from build123d import *

# Parameters (mm, degrees)
F0_R     = 11
F1_DEPTH = 7


with BuildPart() as f1:
    # F0 (on Top) → F1 (new body)
    with BuildSketch(Plane.XY):
        with BuildLine():
            ThreePointArc((-10.362367, 34.413892), (-13.196178, 29.675563), (-13.977698, 24.210082))
            ThreePointArc((-13.977698, 24.210082), (-24.891005, 26.119838), (-33.774991, 19.5))
            ThreePointArc((-33.774991, 19.5), (-35.570661, 13.994279), (-34.984488, 8.232873))
            ThreePointArc((-34.984488, 8.232873), (-32.29788, 3.409556), (-27.955395, 0))
            ThreePointArc((-27.955395, 0), (-35.065946, -8.496324), (-33.774991, -19.5))
            ThreePointArc((-33.774991, -19.5), (-29.904732, -23.807957), (-24.622121, -26.181019))
            ThreePointArc((-24.622121, -26.181019), (-19.101702, -26.266007), (-13.977698, -24.210082))
            ThreePointArc((-13.977698, -24.210082), (-10.174941, -34.616162), (0, -39))
            ThreePointArc((0, -39), (5.665929, -37.802236), (10.362367, -34.413892))
            ThreePointArc((10.362367, -34.413892), (13.196178, -29.675563), (13.977698, -24.210082))
            ThreePointArc((13.977698, -24.210082), (24.891005, -26.119838), (33.774991, -19.5))
            ThreePointArc((33.774991, -19.5), (35.570661, -13.994279), (34.984488, -8.232873))
            ThreePointArc((34.984488, -8.232873), (32.29788, -3.409556), (27.955395, 0))
            ThreePointArc((27.955395, 0), (35.065946, 8.496324), (33.774991, 19.5))
            ThreePointArc((33.774991, 19.5), (29.904732, 23.807957), (24.622121, 26.181019))
            ThreePointArc((24.622121, 26.181019), (19.101702, 26.266007), (13.977698, 24.210082))
            ThreePointArc((13.977698, 24.210082), (10.174941, 34.616162), (0, 39))
            ThreePointArc((0, 39), (-5.665929, 37.802236), (-10.362367, 34.413892))
        make_face()
        with Locations((-21.650635, -12.5)):
            Circle(F0_R, mode=Mode.SUBTRACT)
        with BuildLine():
            ThreePointArc((-6.30476, -12.5), (-7, -12.875644), (-7.672937, -13.289918))
            ThreePointArc((-7.672937, -13.289918), (-7.650635, -12.5), (-7.672937, -11.710082))
            ThreePointArc((-7.672937, -11.710082), (-7, -12.124356), (-6.30476, -12.5))
        make_face(mode=Mode.SUBTRACT)
        with Locations((0, -25)):
            Circle(F0_R, mode=Mode.SUBTRACT)
        with BuildLine():
            ThreePointArc((7.672937, -11.710082), (7.650635, -12.5), (7.672937, -13.289918))
            ThreePointArc((7.672937, -13.289918), (7, -12.875644), (6.30476, -12.5))
            ThreePointArc((6.30476, -12.5), (7, -12.124356), (7.672937, -11.710082))
        make_face(mode=Mode.SUBTRACT)
        with Locations((21.650635, -12.5)):
            Circle(F0_R, mode=Mode.SUBTRACT)
        with Locations((-21.650635, 12.5)):
            Circle(F0_R, mode=Mode.SUBTRACT)
        with BuildLine():
            ThreePointArc((-15.345875, 0), (-14.650635, 0.375644), (-13.977698, 0.789918))
            ThreePointArc((-13.977698, 0.789918), (-14, 0), (-13.977698, -0.789918))
            ThreePointArc((-13.977698, -0.789918), (-14.650635, -0.375644), (-15.345875, 0))
        make_face(mode=Mode.SUBTRACT)
        with BuildLine():
            ThreePointArc((-7.672937, 11.710082), (-7.650635, 12.5), (-7.672937, 13.289918))
            ThreePointArc((-7.672937, 13.289918), (-7, 12.875644), (-6.30476, 12.5))
            ThreePointArc((-6.30476, 12.5), (-7, 12.124356), (-7.672937, 11.710082))
        make_face(mode=Mode.SUBTRACT)
        Circle(F0_R, mode=Mode.SUBTRACT)
        with BuildLine():
            ThreePointArc((13.977698, -0.789918), (14, 0), (13.977698, 0.789918))
            ThreePointArc((13.977698, 0.789918), (14.650635, 0.375644), (15.345875, 0))
            ThreePointArc((15.345875, 0), (14.650635, -0.375644), (13.977698, -0.789918))
        make_face(mode=Mode.SUBTRACT)
        with BuildLine():
            ThreePointArc((6.30476, 12.5), (7, 12.875644), (7.672937, 13.289918))
            ThreePointArc((7.672937, 13.289918), (7.650635, 12.5), (7.672937, 11.710082))
            ThreePointArc((7.672937, 11.710082), (7, 12.124356), (6.30476, 12.5))
        make_face(mode=Mode.SUBTRACT)
        with Locations((21.650635, 12.5)):
            Circle(F0_R, mode=Mode.SUBTRACT)
        with Locations((0, 25)):
            Circle(F0_R, mode=Mode.SUBTRACT)
        with BuildLine():
            ThreePointArc((-34.984488, 8.232873), (-35.570661, 13.994279), (-33.774991, 19.5))
            Line((-33.774991, 19.5), (-40.018085, 8.686644))
            ThreePointArc((-40.018085, 8.686644), (-39.972979, 8.121164), (-39.428556, 7.961773))
            ThreePointArc((-39.428556, 7.961773), (-37.224068, 8.384953), (-34.984488, 8.232873))
        make_face()
        with BuildLine():
            ThreePointArc((-12.81918, 38.127017), (-11.350452, 36.429465), (-10.362367, 34.413892))
            ThreePointArc((-10.362367, 34.413892), (-5.665929, 37.802236), (0, 39))
            Line((0, 39), (-12.486188, 39))
            ThreePointArc((-12.486188, 39), (-12.953356, 38.678197), (-12.81918, 38.127017))
        make_face()
        with BuildLine():
            ThreePointArc((-24.622121, -26.181019), (-29.904732, -23.807957), (-33.774991, -19.5))
            Line((-33.774991, -19.5), (-27.531897, -30.313356))
            ThreePointArc((-27.531897, -30.313356), (-27.019624, -30.557034), (-26.609375, -30.165244))
            ThreePointArc((-26.609375, -30.165244), (-25.873616, -28.044512), (-24.622121, -26.181019))
        make_face()
        with BuildLine():
            ThreePointArc((26.609375, 30.165244), (25.873616, 28.044512), (24.622121, 26.181019))
            ThreePointArc((24.622121, 26.181019), (29.904732, 23.807957), (33.774991, 19.5))
            Line((33.774991, 19.5), (27.531897, 30.313356))
            ThreePointArc((27.531897, 30.313356), (27.019624, 30.557034), (26.609375, 30.165244))
        make_face()
        with BuildLine():
            ThreePointArc((10.362367, -34.413892), (5.665929, -37.802236), (0, -39))
            Line((0, -39), (12.486188, -39))
            ThreePointArc((12.486188, -39), (12.953356, -38.678197), (12.81918, -38.127017))
            ThreePointArc((12.81918, -38.127017), (11.350452, -36.429465), (10.362367, -34.413892))
        make_face()
        with BuildLine():
            ThreePointArc((39.428556, -7.961773), (37.224068, -8.384953), (34.984488, -8.232873))
            ThreePointArc((34.984488, -8.232873), (35.570661, -13.994279), (33.774991, -19.5))
            Line((33.774991, -19.5), (40.018085, -8.686644))
            ThreePointArc((40.018085, -8.686644), (39.972979, -8.121164), (39.428556, -7.961773))
        make_face()
    extrude(amount=F1_DEPTH)


solid = f1.part
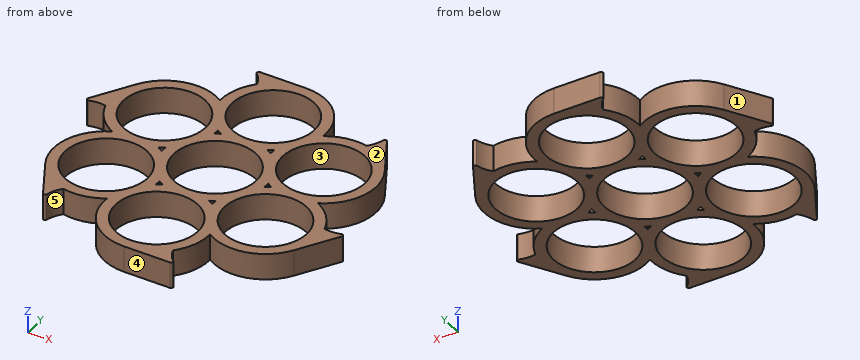
Model file for the job. Use its own axes, mm. Face numbers are marked on the shaded views. A direction names the side the tool comes from. Give positions to 0.01 mm unless a question says otherwise; leave off trailing zeros. Loops run counter-clockwise (first coordinate to the right, second up) from the corner with the lowest first, then second, coordinate; pieces in that order, holes last.
1) Pull direction Y, two halves, no side cores. Call the marked faces 1, 2 and 3: +Y half, -Y half, draft (parallel to the pull), parting line (faces both ways), or undercut.
2) Saw through at D-D (z = 1). Count the separate pieces of the cut face and the enclosed holes in it, plus the area to 3 significant figures.
3) Tool access for the marked faces 4 and 5: list every direction of +Z, -Z, +X, -X, +Y, -Y with a clear straight run to the whole face (end or side of a thin tool).
4) Saw through at A-A (x = -1). Write the cut outline in (y, z).
5) Flat gauge pins, fed straight in: pin 1 Ø17.5 at (x, y) = (21.65, -12.5) entering from -Z; pin 2 Ø2 at (y, z) = (19, 3.5) entering from +X (3 decimals). Where does each tip first touch, or does it go through?
6) Wall check: line 1 (X direction, y = -19.5, z = 3.5) (3 decimals); line 2 (Y direction, x = 3.5, z = 6.75); line 3 (X direction, y = -5, z = 2.5). Give the ranges that are in metal, low to high.
7) Saw through at B-B (x = 19). Write the cut outline in (y, z).
8) Saw through at C-C (y = -3.5). Write the cut outline in (x, z), plus the area to 3 significant figures.
Answer block:
1. face 1: +Y half
1. face 2: draft
1. face 3: undercut
2. separate pieces: 1
2. enclosed holes: 13
2. area: 1,470 mm2
3. face 4: +Z, -Z, +X, -X, -Y
3. face 5: +Z, -Z, -Y
4. outline: (-38.96, 0) - (-35.95, 0) - (-35.95, 7) - (-38.96, 7) - close; (-14.05, 0) - (-10.95, 0) - (-10.95, 7) - (-14.05, 7) - close; (10.95, 0) - (14.05, 0) - (14.05, 7) - (10.95, 7) - close; (35.95, 0) - (39, 0) - (39, 7) - (35.95, 7) - close
5. pin 1: passes through
5. pin 2: stops at x = 34.525
6. line 1: x = -33.775 to -30.136, -13.165 to -9.526, 9.526 to 13.165, 30.136 to 33.775
6. line 2: y = -39 to -35.43, -14.57 to -10.43, 10.43 to 14.57, 35.43 to 38.56
6. line 3: x = -33.47 to -29.7, -13.6 to -9.8, 9.8 to 13.6, 29.7 to 33.47
7. outline: (-26.25, 0) - (-23.18, 0) - (-23.18, 7) - (-26.25, 7) - close; (-1.82, 0) - (1.82, 0) - (1.82, 7) - (-1.82, 7) - close; (23.18, 0) - (26.25, 0) - (26.25, 7) - (23.18, 7) - close
8. outline: (-32.37, 0) - (-27.98, 0) - (-27.98, 7) - (-32.37, 7) - close; (-15.33, 0) - (-10.43, 0) - (-10.43, 7) - (-15.33, 7) - close; (10.43, 0) - (15.33, 0) - (15.33, 7) - (10.43, 7) - close; (27.98, 0) - (32.37, 0) - (32.37, 7) - (27.98, 7) - close
8. area: 130 mm2
